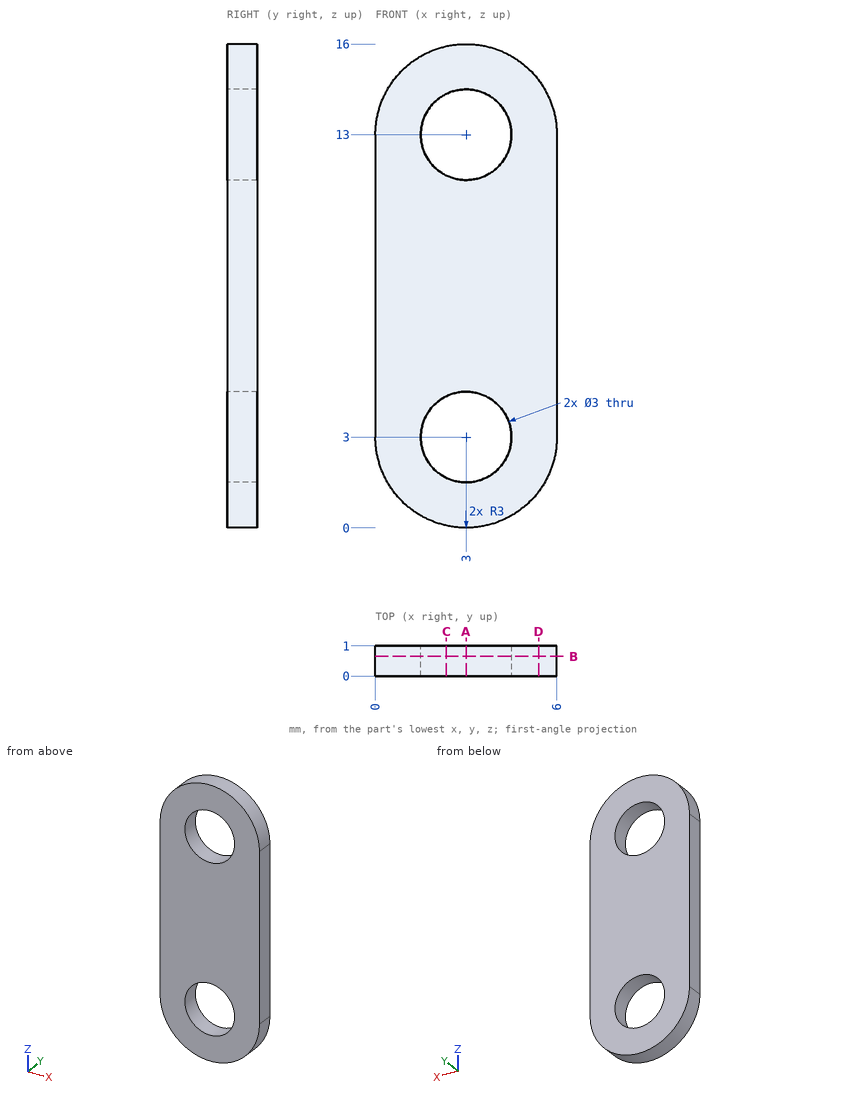
Check sheet for the drawn part. Datum: minimum x, y, z corner. Units: mm. Coordinates: 2 decimals unless noted, no trailing zeros. Order: outer loops, then holes, each group sorted by start corner. A loop starts at its lowest first (then second) coordinate and runs counter-clockwise, first axis right, second up. Notation, with made-up numbers: (22, 81.25) - (28, 81.25) arc R20 cw to (28, 91.25) - close; hole circle Ø7 at (64, 47). An arc over 180 degrees is marked (long way). Return JSON: item names as keys, results as strings.
(1) Section check A-A, the plane x = 3. Record the cut outline in (y, z).
Filled sheet:
{"outline": "(0, 0) - (1, 0) - (1, 1.5) - (0, 1.5) - close; (0, 4.5) - (1, 4.5) - (1, 11.5) - (0, 11.5) - close; (0, 14.5) - (1, 14.5) - (1, 16) - (0, 16) - close"}
(2) Section check D-D, the plane x = 5.4. Record the cut outline in (y, z).
Filled sheet:
{"outline": "(0, 1.2) - (1, 1.2) - (1, 14.8) - (0, 14.8) - close"}
(3) Section check C-C, the plane x = 2.35. Record the cut outline in (y, z), and give its area (3 significant figures).
Filled sheet:
{"outline": "(0, 0.07) - (1, 0.07) - (1, 1.65) - (0, 1.65) - close; (0, 4.35) - (1, 4.35) - (1, 11.65) - (0, 11.65) - close; (0, 14.35) - (1, 14.35) - (1, 15.93) - (0, 15.93) - close", "area": "10.5 mm^2"}
(4) Thickness scan on line 1 along X through (y, z) = (0.25, 3); line 2 along Z through (x, y) = (3, 0.45); line 3 along Z through (x, y) = (2.1, 0.55). Record the ranges inside material, lowest first.
Filled sheet:
{"line 1": "x = 0 to 1.5, 4.5 to 6", "line 2": "z = 0 to 1.5, 4.5 to 11.5, 14.5 to 16", "line 3": "z = 0.14 to 1.8, 4.2 to 11.8, 14.2 to 15.86"}
(5) Go/stop test with a flat-tipped pin: pin 1 (1.5 mm diameter, centred on x = 3, z = 13.5, fed in from -Y). Record where the tip stops, or that it passes through.
Filled sheet:
{"pin 1": "passes through"}
(6) Section check B-B, the plane y = 0.65. Record the cut outline in (x, z), and give its area (3 significant figures).
Filled sheet:
{"outline": "(0, 3) arc R3 ccw to (6, 3) - (6, 13) arc R3 ccw to (0, 13) - close; hole circle Ø3 at (3, 3); hole circle Ø3 at (3, 13)", "area": "74.1 mm^2"}
